Geometry: see drawing. Coordinates: mm, zero at the bounding-box minimum. Give positions to 0.01 mm unless a question says otherwise; leave off trailing zeros. Loops run counter-clockwise (first coordinate to the right, second up) from the corner with the lowest first, then second, coordinate; pieces in that order, holes last. Notation, with made-up numbers: M -6.5,52 L -0.5,52 A9 cw -0.5,59 Z; hole C 24.5,-3.5 d6. An arc over 180 degrees is marked long. Put each result on its own line as item: value.
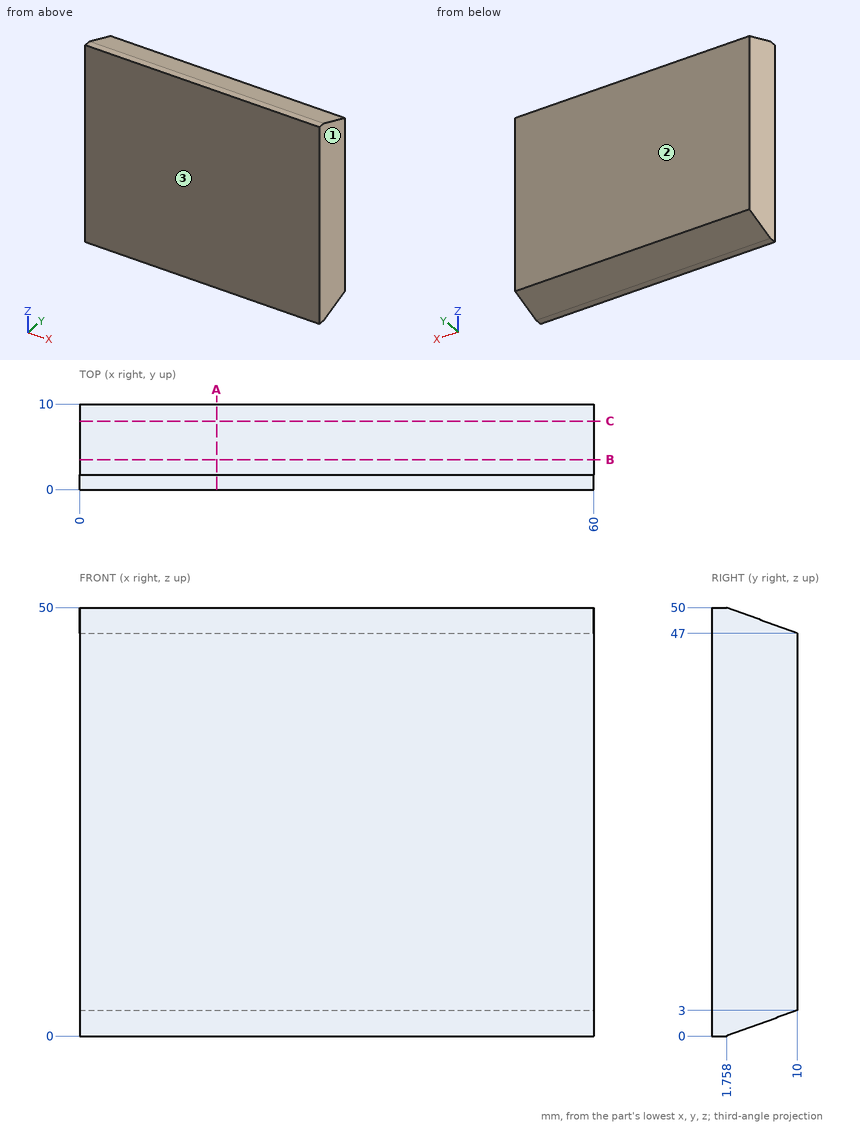
1. Section query C-C (y = 8). Output: boundary loops of the cut face in (x, z), plus the area to 3 significant figures.
Found:
outline: M 0,2.27 L 60,2.27 L 60,47.73 L 0,47.73 Z
area: 2,730 mm^2
2. Contact query for flat-ended pins moving along their axis: P1, Ø2, axis at x = 35, y = 8, coming from the +Z side; P2, Ø4, axis at x = 42.5, y = 4.5, coming from the +Z side. Output: stop coordinate, or through.
Found:
P1: z = 48.09
P2: z = 49.73
3. Draft query along Y for the marked faces 1, 2 and 3. Return one class per face: pulls with the +Y half, pulls with the -Y half, needs draft (parallel to the pull), parting line crosses it, or undercut.
Found:
face 1: needs draft
face 2: pulls with the +Y half
face 3: pulls with the -Y half
4. Material intervals for line 1 (Z direction, x = 50.5, y = 5.25); line 2 (Z direction, x = 32, y = 4) (1 decimal), sorted ascending. Write a range as from..to.
Found:
line 1: 1.27..48.73
line 2: 0.8..49.2
5. Section query B-B (y = 3.5). Output: boundary loops of the cut face in (x, z) (1 decimal), plus the area to 3 significant figures.
Found:
outline: M 0,0.6 L 60,0.6 L 60,49.4 L 0,49.4 Z
area: 2,920 mm^2
6. Section query A-A (x = 16). Output: boundary loops of the cut face in (y, z), plus the area to 3 significant figures.
Found:
outline: M 0,0 L 1.76,0 L 10,3 L 10,47 L 1.76,50 L 0,50 Z
area: 475 mm^2
